Could you check a few things on this drawing? It's one solid part, dimensions in mm from its lowest x, y, z. A direction names the side the tool comes from. Give positions to 0.01 mm unless a question says otherwise; leave off trailing zeros. Loops run counter-clockwise (first coordinate to the right, second up) from the corner with the lowest first, then second, coordinate; pieces in that order, holes last. Notation, with made-up numbers: (46, 26) - (91, 26) arc R25 ccw to (91, 51) - close; hole circle Ø6 at (-6.75, 5.5). An arc over 180 degrees is marked (long way). Use a Markdown table: item, result.
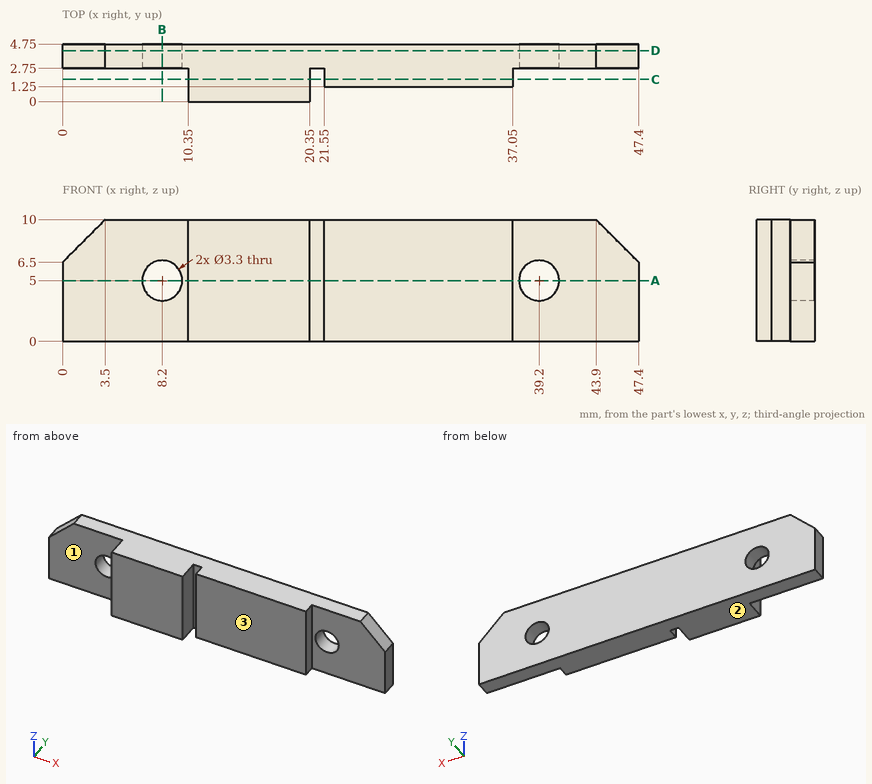
(1) On a 3-axis mill with a long thin cutter (end or side, diameter ignored), from which of +Z, -Z, +X, -X, +Y, -Y can I reach the whole of each face in a straight line? I mean the marked faces 1, 2 and 3. Say none if no direction works.
A:
| item | result |
|---|---|
| face 1 | +Z, -Z, -X, -Y |
| face 2 | -Z, +X, -X, +Y, -Y |
| face 3 | +Z, -Z, +X, -Y |
(2) Suppose I cut it at C-C on y = 1.85. Write out the boundary of the cut face in (x, z).
A:
| item | result |
|---|---|
| outline | (10.35, 0) - (20.35, 0) - (20.35, 10) - (10.35, 10) - close; (21.55, 0) - (37.05, 0) - (37.05, 10) - (21.55, 10) - close |
(3) Suppose I cut it at D-D on y = 4.2. Write out the boundary of the cut face in (x, z).
A:
| item | result |
|---|---|
| outline | (0, 0) - (47.4, 0) - (47.4, 6.5) - (43.9, 10) - (3.5, 10) - (0, 6.5) - close; hole circle Ø3.3 at (8.2, 5); hole circle Ø3.3 at (39.2, 5) |
(4) Suppose I cut it at B-B on x = 8.2. Write out the boundary of the cut face in (y, z).
A:
| item | result |
|---|---|
| outline | (2.75, 0) - (4.75, 0) - (4.75, 3.35) - (2.75, 3.35) - close; (2.75, 6.65) - (4.75, 6.65) - (4.75, 10) - (2.75, 10) - close |
(5) Suppose I cut it at A-A on z = 5. Write out the boundary of the cut face in (x, y).
A:
| item | result |
|---|---|
| outline | (0, 2.75) - (6.55, 2.75) - (6.55, 4.75) - (0, 4.75) - close; (9.85, 2.75) - (10.35, 2.75) - (10.35, 0) - (20.35, 0) - (20.35, 2.75) - (21.55, 2.75) - (21.55, 1.25) - (37.05, 1.25) - (37.05, 2.75) - (37.55, 2.75) - (37.55, 4.75) - (9.85, 4.75) - close; (40.85, 2.75) - (47.4, 2.75) - (47.4, 4.75) - (40.85, 4.75) - close |
(6) If I drill on line 1 (Z direction, x = 8.2, y = 3.9); line 2 (X direction, y = 2.2, z = 4); line 3 (X direction, y = 4.4, z = 6.5), over which ranges is the centre line in solid material (lowest first)?
A:
| item | result |
|---|---|
| line 1 | 0 to 3.35, 6.65 to 10 |
| line 2 | 10.35 to 20.35, 21.55 to 37.05 |
| line 3 | 0 to 7.51, 8.89 to 38.51, 39.89 to 47.4 |
(7) Will these pins go through, and if not, where does the flat tip stop? pin 1 (2 mm diameter, centred on y = 1.5, z = 5, fed in from -X); pin 2 (1.4 mm diameter, centred on y = 1.5, z = 4, fed in from +X).
A:
| item | result |
|---|---|
| pin 1 | x = 10.35 |
| pin 2 | x = 37.05 |
